Study the drawing (mm; zero at the part's minimum x, y, z) and answer. A direction names the side the tool comes from. Coordinates: 2 decimals unless noted, no trailing zeros. Loops run counter-clockwise (first coordinate to the right, second up) from the corner with the lowest first, then second, coordinate; pieces in that order, holes last. Notation, with made-up numbers: (40, 13.5) -> (65, 13.5) arc R26 ccw to (65, 28.5) -> close; hole circle Ø8 at (-9, -29). An arc over 180 degrees is marked (long way). Answer as a JSON object with one key per item and string values. Group by question number.
Q1. For the marked faces 5, 6 and 7, determine the directions among +Z, -Z, +X, -X, +Y, -Y from which every point of the face is accessible in a straight line to the end or side of a thin tool.
Q2. The part is cut by section A-A on y = 17.5. Write down the section's boundary in (x, z).
Q3. Straight lines are drawn through the part: line 1 along Z through (x, y) = (12.5, 11.25); line 2 along X through (y, z) = (0.35, 24.1); line 3 along X through (y, z) = (0.45, 21.6). For each, find the intervals that lie inside material, in ascending order. Write a range as [from, to].
Q4. Determine the mould class of the marked faces 1, 2, 3 and 4 for opening direction X: released by +X, released by -X, zero draft, split by the parting line, or undercut.
Q5. The part is cut by section C-C on y = 3.5. Write down the section's boundary in (x, z), and give its area (3 significant figures).
Q6. The part is cut by section B-B on z = 26.6. Write down the section's boundary in (x, y).
Q7. The part is cut by section D-D on x = 4.5. Write down the section's boundary in (y, z), and give its area (3 significant figures).
Q8. Each of these flat-tipped pins is pushed along its axis until it touches: P1, Ø8, axis at y = 6.5, z = 17, coming from the -X side; P2, Ø1.1, axis at y = 0.5, z = 24.5, coming from the -X side; P3, Ø1.5, axis at x = 3.5, z = 12.5, coming from the +Y side; P4, Ø1.2, axis at x = 12, z = 24.1, coming from the -Y side. Where does it stop, or does it pass through?
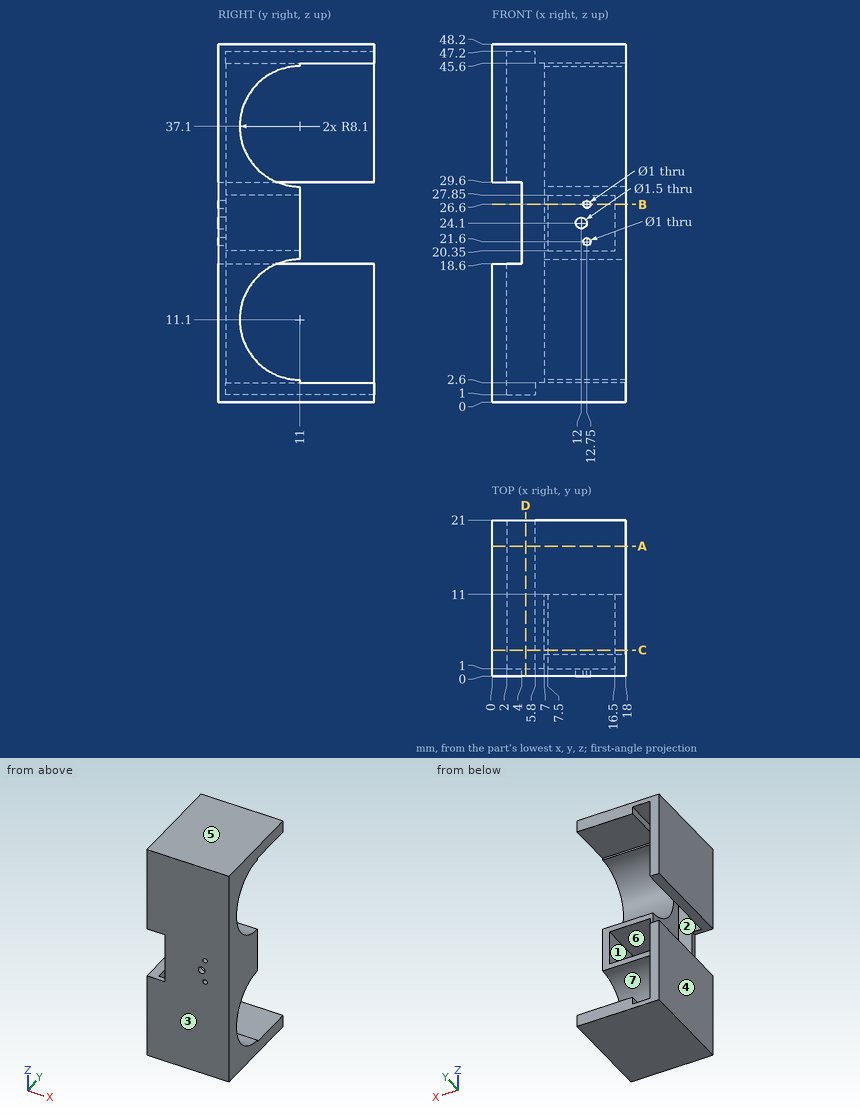
Final values:
{
 "1": {"face 5": "+Z, +X, -X, +Y, -Y", "face 6": "+Y", "face 7": "+X, +Y"},
 "2": {"outline": "(0, 0) -> (18, 0) -> (18, 2.6) -> (5.8, 2.6) -> (5.8, 1) -> (2, 1) -> (2, 18.6) -> (0, 18.6) -> close; (0, 29.6) -> (2, 29.6) -> (2, 47.2) -> (5.8, 47.2) -> (5.8, 45.6) -> (18, 45.6) -> (18, 48.2) -> (0, 48.2) -> close"},
 "3": {"line 1": "z = [0, 2.6], [45.6, 48.2]", "line 2": "x = [4, 11.25], [12.75, 18]", "line 3": "x = [4, 12.25], [13.25, 18]"},
 "4": {"face 1": "undercut", "face 2": "undercut", "face 3": "zero draft", "face 4": "released by -X"},
 "5": {"outline": "(0, 0) -> (18, 0) -> (18, 8.04) -> (7, 8.04) -> (7, 2.6) -> (5.8, 2.6) -> (5.8, 1) -> (2, 1) -> (2, 18.6) -> (0, 18.6) -> close; (0, 29.6) -> (2, 29.6) -> (2, 47.2) -> (5.8, 47.2) -> (5.8, 45.6) -> (7, 45.6) -> (7, 40.16) -> (18, 40.16) -> (18, 48.2) -> (0, 48.2) -> close; (7, 14.16) -> (18, 14.16) -> (18, 34.04) -> (7, 34.04) -> close; hole (7.5, 20.35) -> (16.5, 20.35) -> (16.5, 27.85) -> (7.5, 27.85) -> close", "area": "416 mm2"},
 "6": {"outline": "(4, 0) -> (12.25, 0) -> (12.25, 1) -> (7.5, 1) -> (7.5, 11) -> (7, 11) -> (7, 1) -> (4, 1) -> close; (13.25, 0) -> (18, 0) -> (18, 11) -> (16.5, 11) -> (16.5, 1) -> (13.25, 1) -> close"},
 "7": {"outline": "(0, 0) -> (21, 0) -> (21, 1) -> (1, 1) -> (1, 47.2) -> (21, 47.2) -> (21, 48.2) -> (0, 48.2) -> close", "area": "88.2 mm2"},
 "8": {"P1": "stops at x = 0", "P2": "stops at x = 4", "P3": "stops at y = 1", "P4": "passes through"}
}
